Input: part model. Units: mm. Frame: model coordinates. Face numbers are marked on the shaded views. A direction names the side the tool comes from. Coordinates: 2 decimals unless noted, no trailing zeros. Write each loop counter-clockwise with the first axis right and the second up, starting at its lowest first coordinate (ties: lowest second). Pieces come first, ordered by that corner, then holes. Notation, with made-up numbers: (71, 19.25) - (114, 19.25) arc R23 ccw to (114, 54.25) - close; hole circle Ø11 at (-38.75, 14). An arc over 180 degrees is marked (long way). One line per question, with ' | ' between items. Start each with the question number.
1) Section query D-D on x = -196.5. Return loops of the section in (y, z).
2) Section query A-A on y = -8. Return loops of the section in (x, z), and give its area (3 significant figures).
3) First-contact query: P1, Ø3, axis at x = -205.5, z = 7, coming from the +Y side; P2, Ø4, axis at x = -214, z = 4, coming from the -Y side. Flat tips, straight axial feed; report the tip coordinate or a pass-through.
4) Section query C-C on y = 12. Return loops of the section in (x, z), and give its area (3 significant figures).
5) Line query: line 1 (Y direction, x = -183, z = 9.25); line 2 (X direction, y = 8, z = 2.5); line 3 (X direction, y = -10, z = 6.5). Output: solid intervals per line, ascending.
6) Section query B-B on z = 5.75. Return loops of the section in (x, y), and give its area (3 significant figures).
7) Reachability of the marked faces 3, 4 and 5 from +Z, -Z, +X, -X, +Y, -Y: full face, straight path, thin tool, end or side. Return the list, or none.
8) Draft query along X for the marked faces 1 and 2. Return one class per face: released by +X, released by -X, zero draft, split by the parting line, or undercut.
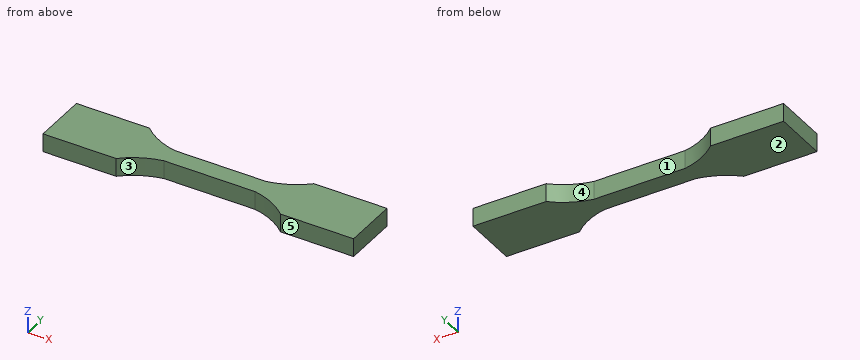
```python
from build123d import *

# Parameters (mm, degrees)
F1_DEPTH = 10
F2_ANGLE = 90


with BuildPart() as f1:
    # F0 (on Top) → F1 (new body)
    with BuildSketch(Plane.XY):
        with BuildLine():
            Line((-15, -85), (15, -85))
            Line((15, -85), (15, -45))
            ThreePointArc((15, -45), (8.5740404346, -35.7129797827), (5, -25))
            Line((5, -25), (5, 25))
            ThreePointArc((5, 25), (8.5740404346, 35.7129797827), (15, 45))
            Line((15, 45), (15, 85))
            Line((15, 85), (-15, 85))
            Line((-15, 85), (-15, 45))
            ThreePointArc((-15, 45), (-8.5740404346, 35.7129797827), (-5, 25))
            Line((-5, 25), (-5, -25))
            ThreePointArc((-5, -25), (-8.5740404346, -35.7129797827), (-15, -45))
            Line((-15, -45), (-15, -85))
        make_face()
    extrude(amount=F1_DEPTH)


with BuildPart() as f1_1:
    # F2: moved
    add(f1.part.rotate(Axis((-15, -85, 5), (0, 0, -1)), F2_ANGLE))


with BuildPart() as f1_2:
    # F3: moved
    add(f1_1.part.moved(Location((-70, 100, 0))))


with BuildPart() as f1_3:
    # F4: moved
    add(f1_2.part.moved(Location((-200, 0, 0))))


solid = f1_3.part
```
Answer key:
1) outline: (-5, 0) - (5, 0) - (5, 10) - (-5, 10) - close
2) outline: (-285, 0) - (-234.52, 0) - (-234.52, 10) - (-285, 10) - close; (-165.48, 0) - (-115, 0) - (-115, 10) - (-165.48, 10) - close | area: 1,010 mm²
3) P1: y = 5 | P2: y = -5
4) outline: (-285, 0) - (-241.35, 0) - (-241.35, 10) - (-285, 10) - close; (-158.65, 0) - (-115, 0) - (-115, 10) - (-158.65, 10) - close | area: 873 mm²
5) line 1: -5 to 5 | line 2: -285 to -234.52, -165.48 to -115 | line 3: -285 to -238.32, -161.68 to -115
6) outline: (-285, -15) - (-245, -15) arc R40 cw to (-225, -5) - (-175, -5) arc R40 cw to (-155, -15) - (-115, -15) - (-115, 15) - (-155, 15) arc R40 cw to (-175, 5) - (-225, 5) arc R40 cw to (-245, 15) - (-285, 15) - close | area: 3,600 mm²
7) face 3: +Z, -Z, -Y | face 4: +Z, -Z, +Y | face 5: +Z, -Z, +X, -X, -Y
8) face 1: undercut | face 2: zero draft
